Autodesk Inventor part; units mm, degrees
ref_plane "YZ Plane" through (0, 0, 0) normal (1, 0, 0) x (0, 1, 0)
ref_plane "XZ Plane" through (0, 0, 0) normal (0, 1, 0) x (-1, 0, 0)
ref_plane "XY Plane" through (0, 0, 0) normal (0, 0, 1) x (1, 0, 0)
sketch "Sketch1" plane through (0, 0, 0) normal (0, 1, 0) x (-1, 0, 0)
  line L0 (0, 0) -> (47.635, 0)
  line L1 (47.635, 0) -> (47.635, -52.715)
  line L2 (47.635, -52.715) -> (0, -52.715)
  line L3 (0, -52.715) -> (0, 0)
  circle A0 centre (45.725, -1.91) radius 2.1
  circle A1 centre (45.725, -50.805) radius 2.1
  circle A2 centre (1.91, -1.91) radius 2.1
  circle A3 centre (1.91, -50.805) radius 2.1
  line L4 (47.635, 0) -> (51.445, 0)
  line L5 (51.445, 0) -> (51.445, -52.715)
  line L6 (51.445, -52.715) -> (47.635, -52.715)
  line L7 (47.635, -52.715) -> (47.635, 0)
  line L8 (0, 0) -> (-3.81, 0)
  line L9 (-3.81, 0) -> (-3.81, -56.525)
  line L10 (-3.81, -56.525) -> (0, -56.525)
  line L11 (0, -56.525) -> (0, 0)
  line L12 (51.445, -52.715) -> (-6.35, -52.715)
  line L13 (-6.35, -52.715) -> (-6.35, -56.525)
  line L14 (-6.35, -56.525) -> (51.445, -56.525)
  line L15 (51.445, -56.525) -> (51.445, -52.715)
  line L16 (-3.81, 0) -> (51.445, 0)
  line L17 (51.445, 0) -> (51.445, 3.81)
  line L18 (51.445, 3.81) -> (-3.81, 3.81)
  line L19 (-3.81, 3.81) -> (-3.81, 0)
  point P0 (0, -52.715)
  point P1 (0, -51.6779)
  point P2 (0, -49.9321)
  point P3 (0, -2.7829)
  point P4 (0, -1.0371)
  point P5 (-3.81, -77.675)
  point P6 (-3.81, -52.715)
  point P7 (0, -52.715)
  point P8 (1.0371, -52.715)
  point P9 (2.7829, -52.715)
  point P10 (0, -52.715)
  point P11 (0, -56.525)
  point P12 (0, -56.525)
  dimension "d0" = 52.715
  dimension "d1" = 47.635
  dimension "d3" = 4.2
  dimension "d4" = 4.2
  dimension "d6" = 1.91
  dimension "d7" = 1.91
  dimension "d8" = 1.91
  dimension "d9" = 4.2
  dimension "d10" = 4.2
  dimension "d11" = 1.91
  dimension "d12" = 1.91
  dimension "d13" = 1.91
  dimension "d14" = 1.91
  dimension "d15" = 1.91
  dimension "d18" = 3.81
  dimension "d19" = 3.81
  dimension "d20" = 3.81
  dimension "d21" = 3.81
  dimension "d38" = 0
  dimension "d39" = 0
extrude "Extrusion5" add sketch "Sketch1" along normal blind 6 contours L8 L19 L18 L17 L4 L0 A0 A2 | L0 A2 L3 | L3 A2 A3 L12 L9 L8 | L0 A0 L1 A1 L2 A3 L3 A2 | L12 L11 L10 L9 | L3 A3 L2 | L2 A3 A1 L6 L15 L14 L11 | L0 L1 A0 | A0 L1 L4 L5 L6 A1 | L1 L2 A1 picked at (0.2904, -0.2904) picked at (0.2904, -52.4246) picked at (47.3446, -0.2904) picked at (47.3446, -52.4246)
sketch "Sketch6" plane through (0, 6, 0) normal (0, 1, 0) x (1, 0, 0)
  line L0 (-51.445, -3.81) -> (3.81, -3.81)
  line L1 (-51.445, -3.81) -> (-38.745, -3.81)
  line L2 (-38.745, -3.81) -> (-38.745, 8.89)
  line L3 (-38.745, 8.89) -> (-51.445, 8.89)
  line L4 (-51.445, 8.89) -> (-51.445, -3.81)
  line L5 (3.81, 56.525) -> (-51.445, 56.525)
  line L6 (-51.445, 56.525) -> (-38.745, 56.525)
  line L7 (-38.745, 56.525) -> (-38.745, 43.825)
  line L8 (-38.745, 43.825) -> (-51.445, 43.825)
  line L9 (-51.445, 43.825) -> (-51.445, 56.525)
  line L10 (3.81, -3.81) -> (3.81, 56.525)
  line L11 (3.81, 56.525) -> (-8.89, 56.525)
  line L12 (-8.89, 56.525) -> (-8.89, 43.825)
  line L13 (-8.89, 43.825) -> (3.81, 43.825)
  line L14 (3.81, 43.825) -> (3.81, 56.525)
  line L15 (3.81, -3.81) -> (-8.89, -3.81)
  line L16 (-8.89, -3.81) -> (-8.89, 8.89)
  line L17 (-8.89, 8.89) -> (3.81, 8.89)
  line L18 (3.81, 8.89) -> (3.81, -3.81)
  line L19 (3.81, 56.525) -> (-51.445, 56.525)
  line L20 (-51.445, 56.525) -> (-51.445, -3.81)
  line L21 (-51.445, -3.81) -> (3.81, -3.81)
  line L22 (3.81, -3.81) -> (3.81, 56.525)
  circle A0 centre (-1.91, 1.91) radius 2.1
  circle A1 centre (-45.725, 1.91) radius 2.1
  circle A2 centre (-45.725, 50.805) radius 2.1
  circle A3 centre (-1.91, 50.805) radius 2.1
  point P0 (0, 0)
  point P1 (3.81, 8.89)
  dimension "d42" = 12.7
  dimension "d43" = 12.7
  dimension "d44" = 12.7
  dimension "d45" = 12.7
  dimension "d46" = 12.7
  dimension "d47" = 12.7
extrude "Extrusion6" cut sketch "Sketch6" against normal blind 5 contours L2 L3 L20 L8 L7 L5 L12 L13 L10 L17 L16 L0
sketch "Sketch7" plane through (0, 0, 0) normal (0, -1, 0) x (1, 0, 0)
  line L0 (3.81, -56.525) -> (-51.445, -56.525)
  line L1 (3.81, 3.81) -> (3.81, -56.525)
  line L2 (-51.445, 3.81) -> (3.81, 3.81)
  line L3 (-51.445, -56.525) -> (-51.445, 3.81)
  circle A0 centre (-1.91, -1.91) radius 2.1
  circle A1 centre (-45.725, -1.91) radius 2.1
  circle A2 centre (-45.725, -50.805) radius 2.1
  circle A3 centre (-1.91, -50.805) radius 2.1
  line L4 (-8.89, 3.81) -> (3.81, 3.81)
  line L5 (3.81, 3.81) -> (-51.445, 3.81)
  line L6 (-51.445, 3.81) -> (-51.445, 6.35)
  line L7 (-51.445, 6.35) -> (3.81, 6.35)
  line L8 (3.81, 6.35) -> (3.81, 3.81)
  line L9 (-51.445, 6.35) -> (-53.985, 6.35)
  line L10 (-53.985, 6.35) -> (-53.985, -56.525)
  line L11 (-53.985, -56.525) -> (-51.445, -56.525)
  line L12 (-51.445, -56.525) -> (-51.445, 6.35)
  line L13 (-53.985, -56.525) -> (3.81, -56.525)
  line L14 (3.81, -56.525) -> (3.81, -59.065)
  line L15 (3.81, -59.065) -> (-53.985, -59.065)
  line L16 (-53.985, -59.065) -> (-53.985, -56.525)
  line L17 (3.81, -59.065) -> (6.35, -59.065)
  line L18 (6.35, -59.065) -> (6.35, 5.08)
  line L19 (6.35, 5.08) -> (3.81, 5.08)
  line L20 (3.81, 5.08) -> (3.81, -59.065)
  line L21 (6.35, 5.08) -> (3.81, 5.08)
  line L22 (3.81, 5.08) -> (3.81, 6.35)
  line L23 (3.81, 6.35) -> (6.35, 6.35)
  line L24 (6.35, 6.35) -> (6.35, 5.08)
  point P0 (0, 0)
  dimension "d50" = 2.54
  dimension "d51" = 2.54
  dimension "d52" = 2.54
  dimension "d53" = 2.54
extrude "Extrusion7" add sketch "Sketch7" against normal blind 8 contours L14 L15 L16 L11 L0 | L1 L8 L19 L18 L17 L14 | L11 L10 L9 L6 L3 | L2 L6 L7 L8 | L8 L23 L24 L19
sketch "Sketch8" plane through (0, 8, 0) normal (0, 1, 0) x (1, 0, 0)
  line L0 (-53.985, -6.35) -> (6.35, -6.35)
  line L1 (6.35, -6.35) -> (6.35, 59.065)
  line L2 (6.35, 59.065) -> (-53.985, 59.065)
  line L3 (-53.985, 59.065) -> (-53.985, -6.35)
  line L4 (3.81, 56.525) -> (3.81, -3.81)
  line L5 (3.81, -3.81) -> (-51.445, -3.81)
  line L6 (-51.445, -3.81) -> (-51.445, 56.525)
  line L7 (-51.445, 56.525) -> (3.81, 56.525)
  circle A0 centre (-1.91, 50.805) radius 2.1
  line L8 (-1.91, 50.805) -> (-10.17, 50.805)
  line L9 (-10.17, 50.805) -> (-10.17, 48.127)
  line L10 (-10.17, 48.127) -> (-1.91, 48.127)
  line L11 (-1.91, 48.127) -> (-1.91, 50.805)
  line L12 (6.35, 59.065) -> (-53.985, 59.065)
  line L13 (-10.17, 48.127) -> (-22.87, 48.127)
  line L14 (-22.87, 48.127) -> (-22.87, 59.065)
  line L15 (-22.87, 59.065) -> (-10.17, 59.065)
  line L16 (-10.17, 59.065) -> (-10.17, 48.127)
  point P0 (0, 0)
  point P1 (-10.17, 56.525)
  point P2 (-22.87, 56.525)
  dimension "d56" = 8.26
  dimension "d57" = 12.7
extrude "Extrusion8" cut sketch "Sketch8" against normal blind 8 contours L2 L16 L7 L14
properties part number "PCB_REMOTE_Holder_"
Can you work these out from the model? Positions are in its coordinate system, mm. A direction names the side the tool comes from. Round coordinates to 2 decimals unless told otherwise and drop trailing zeros. Loops run counter-clockwise (first coordinate to the right, second up) from the corner with the lowest first, then second, coordinate; pieces in that order, holes last. Notation, with made-up numbers: (24, -5) - (33, -5) arc R26 cw to (33, 12) - close; hole circle Ø4 at (15, -14). An arc over 180 degrees is marked (long way). Answer in a Markdown table with one row per item. Add a question column.
Q1. I want a section at A-A on x = -1.91. List the corners of the cut face in (y, z) for me (3 decimals).
Q2. I need wall thicknesses on L1, parallel to X at y = 3.25, z = -1.91 (3 decimals); L2, parallel to Z at x = -1.91, y = 4.6 (3 decimals); L3, parallel to X at y = 5.5, z = -23.5 (3 decimals). Which ranges of each line are inside material? Lowest first, please.
Q3. I want a section at D-D on x = -26.5. List the corners of the cut face in (y, z) for me (3 decimals).
Q4. I want a section at B-B on z = -1.91. List the corners of the cut face in (x, y) for me (3 decimals), and give its area (3 significant figures).
Q5. For pin 1 Ø4 at (x, z) = (-46, -51.5) entering from +Y; pin 2 Ø2 at (x, z) = (-15, -15.5) entering from +Y, each with a flat end and sliding along its axis, tell me the tip position at first contact or that it passes through.
Q6. We'd pull the mould along X, two halves only. Please class faces 4 (the flat face through (-2, 4, -59.065)), 5 (the flat face through (-53.985, 4, -27)), 6 (the cylindrical face through (-0.244, 2.958, -0.632)): pulls with the +X half, pulls with the -X half, needs draft (parallel to the pull), parting line crosses it, or undercut.
Q7. Which directions (+Z, -Z, +X, -X, +Y, -Y) give clear straight access to the entire face, cutting with the end or side of a thin tool? Please do faces 1 (the flat face through (-23, 4, 6.35)), 2 (the flat face through (-10.17, 4, -58)), 3 (the flat face through (-8.89, 4, -50)).
Q8. I want a section at C-C on z = -17. List the corners of the cut face in (x, y) for me (3 decimals).
A:
| question | item | result |
|---|---|---|
| 1 | outline | (0, -59.065) - (8, -59.065) - (8, -56.525) - (6, -56.525) - (6, -52.905) - (0, -52.905) - close; (0, -48.705) - (6, -48.705) - (6, -43.825) - (1, -43.825) - (1, -8.89) - (6, -8.89) - (6, -4.01) - (0, -4.01) - close; (0, 0.19) - (6, 0.19) - (6, 3.81) - (8, 3.81) - (8, 6.35) - (0, 6.35) - close |
| 2 | L1 | -53.985 to -47.825, -43.625 to -38.745, -8.89 to -4.01, 0.19 to 6.35 |
| 2 | L2 | -59.065 to -52.905, -48.705 to -43.825, -8.89 to -4.01, 0.19 to 6.35 |
| 2 | L3 | -53.985 to -51.445, 3.81 to 6.35 |
| 3 | outline | (0, -59.065) - (8, -59.065) - (8, -56.525) - (1, -56.525) - (1, 3.81) - (8, 3.81) - (8, 6.35) - (0, 6.35) - close |
| 4 | outline | (-53.985, 0) - (-47.825, 0) - (-47.825, 6) - (-51.445, 6) - (-51.445, 8) - (-53.985, 8) - close; (-43.625, 0) - (-4.01, 0) - (-4.01, 6) - (-8.89, 6) - (-8.89, 1) - (-38.745, 1) - (-38.745, 6) - (-43.625, 6) - close; (0.19, 0) - (6.35, 0) - (6.35, 8) - (3.81, 8) - (3.81, 6) - (0.19, 6) - close |
| 4 | area | 172 mm^2 |
| 5 | pin 1 | y = 6 |
| 5 | pin 2 | y = 1 |
| 6 | face 4 | needs draft |
| 6 | face 5 | pulls with the -X half |
| 6 | face 6 | undercut |
| 7 | face 1 | +Z, +X, -X, +Y, -Y |
| 7 | face 2 | -Z, +Y, -Y |
| 7 | face 3 | +Y |
| 8 | outline | (-53.985, 0) - (6.35, 0) - (6.35, 8) - (3.81, 8) - (3.81, 1) - (-51.445, 1) - (-51.445, 8) - (-53.985, 8) - close |
